The listing builds one solid part. Answer for the finished solid, in the listing's coordinates (mm). Face numbers are marked on the shaded views. A direction names the side the tool comes from. Give positions to 0.01 mm unless a question says otherwise; leave off trailing zeros. Order: outer loops, then holes, each group sorted by start corner. A loop starts at its lowest first (then second) coordinate and runs counter-clockwise, first axis right, second up. Notation, with made-up numbers: (8.25, -1.5) - (45.25, -1.5) arc R33 cw to (45.25, 28.5) - close; hole circle Ø4 at (3, -27.75). An arc over 180 degrees is marked (long way). Answer as a JSON object with one key per item and string values. Group by question number.
Q1. A cutting plane is placed at C-C, the plane y = 6. Give the vertices of the cut face in (x, z).
Q2. For the marked faces 1 and 2, determine the directions among +Z, -Z, +X, -X, +Y, -Y from which every point of the face is accessible in a straight line to the end or side of a thin tool.
Q3. Given pin 1 (3 mm diameter, centred on y = 5.5, z = -0.5, fed in from +X); pin 2 (6.5 mm diameter, centred on x = 0, y = 7.5, fed in from -Z); pin 3 (6 mm diameter, centred on x = -9, y = 6, fed in from +Z), each flat-ended and moving along its own axis, determine where each tip first touches the part or whether it passes through.
Q4. The mould has two halves that part along Z. Classify the marked faces 3, 4 and 5: released by +Z, released by -Z, zero draft, split by the parting line, or undercut.
Q5. Consider line 1 (X direction, y = 3, z = 0); line 2 (Z direction, x = -7, y = 1.75); line 3 (X direction, y = 0.5, z = -10). Determine where each line is inside the solid, lowest interval first.
Q6. A cutting plane is placed at A-A, the plane z = 0. Give the vertices of the cut face in (x, y), and give its area (3 significant figures).
Q7. A cutting plane is placed at D-D, the plane z = 7. Give the vertices of the cut face in (x, y).
Q8. A cutting plane is placed at B-B, the plane x = 0. Give the vertices of the cut face in (y, z), and give its area (3 significant figures).
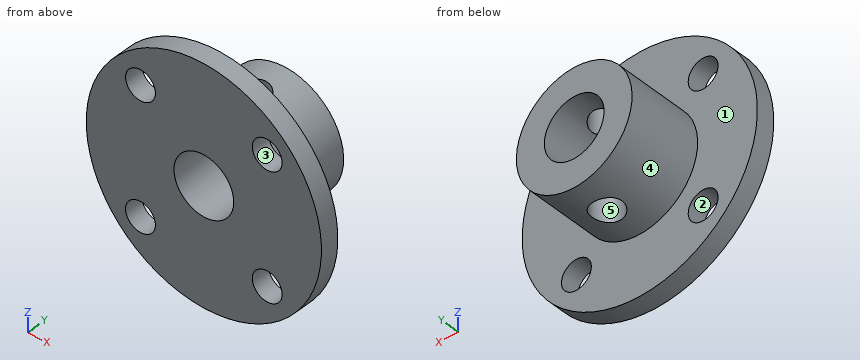
from build123d import *

# Parameters (mm, degrees)
SKETCH1_R               = 15.75
BOSS_EXTRUDE1_DEPTH     = 2.5
SKETCH2_R               = 7.75
BOSS_EXTRUDE2_DEPTH     = 10
SKETCH3_R               = 4
CUT_EXTRUDE1_DEPTH      = 26.541632681
CUT_EXTRUDE2_DEPTH      = 26.541632681
CUT_EXTRUDE2_DEPTH_BACK = 26.541632681
SKETCH4_R               = 2
SKETCH5_R               = 2
CUT_EXTRUDE3_DEPTH      = 26.54163273


with BuildPart() as part:
    # Sketch1 → Boss-Extrude1 (new body)
    with BuildSketch(Plane(origin=(0, 0, 0), x_dir=(1, 0, 0), z_dir=(0, 1, 0))):
        with Locations(Location((0, 0, 0), (0, 0, 270))):
            Circle(SKETCH1_R)
    extrude(amount=BOSS_EXTRUDE1_DEPTH)

    # Sketch2 → Boss-Extrude2 (add)
    with BuildSketch(Plane(origin=(0, 2.5, 0), x_dir=(1, 0, 0), z_dir=(0, 1, 0))):
        with Locations(Location((0, 0, 0), (0, 0, 270))):
            Circle(SKETCH2_R)
    extrude(amount=BOSS_EXTRUDE2_DEPTH)

    # Sketch3 → Cut-Extrude1 (cut, through all)
    with BuildSketch(Plane.XZ):
        with Locations(Location((0, 0, 0), (0, 0, 270))):
            Circle(SKETCH3_R)
    extrude(amount=-CUT_EXTRUDE1_DEPTH, mode=Mode.SUBTRACT)

    # Sketch4 → Cut-Extrude2 (cut, two sides: drawn at the far end of the back side and taken through both)
    with BuildSketch(Plane.XY.offset(-CUT_EXTRUDE2_DEPTH_BACK)):
        with Locations((0, 7.5)):
            Circle(SKETCH4_R)
    extrude(amount=CUT_EXTRUDE2_DEPTH + CUT_EXTRUDE2_DEPTH_BACK, mode=Mode.SUBTRACT)

    # Sketch5 → Cut-Extrude3 (cut, through all)
    with BuildSketch(Plane.XZ):
        with Locations(Location((8.485281374, 8.485281374, 0), (0, 0, 270))):
            Circle(SKETCH5_R)
        with Locations(Location((8.485281374, -8.485281374, 0), (0, 0, 270))):
            Circle(SKETCH5_R)
        with Locations(Location((-8.485281374, -8.485281374, 0), (0, 0, 270))):
            Circle(SKETCH5_R)
        with Locations(Location((-8.485281374, 8.485281374, 0), (0, 0, 270))):
            Circle(SKETCH5_R)
    extrude(amount=-CUT_EXTRUDE3_DEPTH, mode=Mode.SUBTRACT)


solid = part.part
Reply:
{
 "1": {"outline": "(-1.32, -7.64) - (-1.32, -3.77) arc R4 cw to (-1.32, 3.77) - (-1.32, 7.64) arc R7.75 ccw to start; (1.32, -7.64) arc R7.75 ccw to (1.32, 7.64) - (1.32, 3.77) arc R4 cw to (1.32, -3.77) - close"},
 "2": {"face 1": "+Y", "face 2": "+Y, -Y"},
 "3": {"pin 1": "stops at x = 7.75", "pin 2": "stops at z = -7.75", "pin 3": "stops at z = 4.91"},
 "4": {"face 3": "undercut", "face 4": "split by the parting line", "face 5": "zero draft"},
 "5": {"line 1": "x = -7.75 to -4, 4 to 7.75", "line 2": "z = -14.11 to -9.82, -7.15 to 7.15, 9.82 to 14.11", "line 3": "x = -12.17 to -9.79, -7.18 to 7.18, 9.79 to 12.17"},
 "6": {"outline": "(-15.75, 0) - (-4, 0) - (-4, 12.5) - (-7.75, 12.5) - (-7.75, 2.5) - (-15.75, 2.5) - close; (4, 0) - (15.75, 0) - (15.75, 2.5) - (7.75, 2.5) - (7.75, 12.5) - (4, 12.5) - close", "area": "134 mm^2"},
 "7": {"outline": "(-14.11, 0) - (-9.82, 0) - (-9.82, 2.5) - (-14.11, 2.5) - close; (-7.15, 0) - (7.15, 0) - (7.15, 2.5) - (3.33, 2.5) - (3.33, 12.5) - (-3.33, 12.5) - (-3.33, 2.5) - (-7.15, 2.5) - close; (9.82, 0) - (14.11, 0) - (14.11, 2.5) - (9.82, 2.5) - close; hole circle Ø4 at (0, 7.5)"},
 "8": {"outline": "(0, -15.75) - (2.5, -15.75) - (2.5, -7.75) - (5.5, -7.75) - (5.5, -4) - (0, -4) - close; (0, 4) - (5.5, 4) - (5.5, 7.75) - (2.5, 7.75) - (2.5, 15.75) - (0, 15.75) - close; (9.5, -7.75) - (12.5, -7.75) - (12.5, -4) - (9.5, -4) - close; (9.5, 4) - (12.5, 4) - (12.5, 7.75) - (9.5, 7.75) - close", "area": "104 mm^2"}
}
